Design review of the part built by this model. Coordinates are the model's own, in mm. A direction names the side the tool comes from. Coordinates: 2 decimals unless noted, no trailing zeros. Write each loop counter-clockwise with the first axis right and the second up, starting at its lowest first coordinate (ties: lowest second). Pieces come first, ordered by that corner, then holes.
Q1. Add section C-C, the plane y = 6.5. Give the boundary of the cut face in (x, z) (3 decimals).
Q2. To check wall thickness, follow probe 1 along X at (y, z) = (0.4, -12.1); probe 2 along X at (y, z) = (-1, -12.75); probe 3 along X at (y, z) = (2, -10.75). State the ranges of each line that lie inside material, in increasing order.
Q3. Add section D-D, the plane z = -8. Give the boundary of the cut face in (x, y).
Q4. The part is to be moulded in two halves that separate along X. For faces 1 (the face through (9.045, 1.521, -6.024)), 2 (the face through (-4, 2, -11)), 3 (the face through (9.5, 1.5, -7)), say which applies: +X half, -X half, draft (parallel to the pull), parting line (faces both ways), or undercut.
Q5. Add section A-A, the plane z = -5. Give the boundary of the cut face in (x, y) (3 decimals).
Q6. Clearance check with flat-ended pins moving along their axes: pin 1 Ø1.7 at (x, z) = (4, -4.5) entering from -Y; pin 2 Ø3.5 at (x, z) = (-1.5, -13) entering from -Y; pin 3 Ø1.7 at (y, z) = (7, -5.5) entering from +X; pin 4 Ø1.8 at (x, y) = (4, 7) entering from -Z. State where each tip first meets the part, or that it passes through.
Q7. Machinability: for faces 4 (the face through (5, 9.55, -5)), 5 (the face through (3, 6, -3)), 6 (the face through (-1.134, -0.021, -13.578)), 7 (the face through (-3.754, 0.305, -12.941)), 8 (the face through (1.45, 3.64, -14.2)), which of the approach directions +Z, -Z, +X, -X, +Y, -Y give a long, thin tool a straight path to every point of the face, cutting with its end or side? Answer none if there is none.
from build123d import *

# Parameters (mm, degrees)
SKETCH1_W           = 9
SKETCH1_H           = 9
BOSS_EXTRUDE1_DEPTH = 3
SKETCH2_W           = 2.95
SKETCH2_H           = 6
BOSS_EXTRUDE2_DEPTH = 6.1
FILLET1_R           = 3
SKETCH3_R           = 0.975
CUT_EXTRUDE1_DEPTH  = 11.1
CUT_EXTRUDE3_DEPTH  = 21.1
BOSS_EXTRUDE3_START = 4
SKETCH5_R           = 3
BOSS_EXTRUDE3_DEPTH = 4
SKETCH8_R           = 1.55
CUT_EXTRUDE4_DEPTH  = 3
CUT_EXTRUDE5_DEPTH  = 0.5
SKETCH10_W          = 9
SKETCH10_H          = 3
BOSS_EXTRUDE4_DEPTH = 4
SKETCH11_R          = 1
CUT_EXTRUDE6_DEPTH  = 4
CUT_EXTRUDE7_DEPTH  = 4
SKETCH13_W          = 6.1
SKETCH13_H          = 4
BOSS_EXTRUDE7_DEPTH = 7.5
SKETCH16_W          = 1.55
SKETCH16_H          = 4.1
CUT_EXTRUDE9_DEPTH  = 3.2
SKETCH17_W          = 4
SKETCH17_H          = 3
BOSS_EXTRUDE8_DEPTH = 2
SKETCH19_R          = 1.025
CUT_EXTRUDE10_DEPTH = 4
FILLET2_R           = 1


with BuildPart() as part:
    # Sketch1 → Boss-Extrude1 (new body)
    with BuildSketch(Plane(origin=(0, 0, 0), x_dir=(1, 0, 0), z_dir=(0, 1, 0))):
        with Locations((4.5, 4.5)):
            Rectangle(SKETCH1_W, SKETCH1_H)
    extrude(amount=BOSS_EXTRUDE1_DEPTH)

    # Sketch2 → Boss-Extrude2 (add)
    with BuildSketch(Plane(origin=(0, 0, -9), x_dir=(-1, 0, 0), z_dir=(0, 0, -1))):
        with Locations((-7.525, 1.5)):
            Rectangle(SKETCH2_W, SKETCH2_H)
        with Locations((-1.475, 1.5)):
            Rectangle(SKETCH2_W, SKETCH2_H)
    extrude(amount=BOSS_EXTRUDE2_DEPTH)

    # Fillet1
    fillet1_edges = [part.edges().sort_by_distance(p)[0] for p in [
        (1.475, 4.5, -15.1),
        (1.475, -1.5, -15.1),
        (7.525, -1.5, -15.1),
        (7.525, 4.5, -15.1),
    ]]
    fillet(fillet1_edges, radius=FILLET1_R - 0.0001)  # a hair under: the kernel refuses the full size

    # Sketch3 → Cut-Extrude1 (cut)
    with BuildSketch(Plane(origin=(9, 0, 0), x_dir=(0, 0, -1), z_dir=(1, 0, 0))):
        with Locations((12.1, 1.5)):
            Circle(SKETCH3_R)
    extrude(amount=-CUT_EXTRUDE1_DEPTH, mode=Mode.SUBTRACT)

    # Sketch6 → Cut-Extrude3 (cut)
    with BuildSketch(Plane.ZY):
        with BuildLine():
            Line((-12.1, 4.5), (-9, 4.5))
            Line((-9, 4.5), (-9, 3))
            Line((-9, 3), (-9.501923789, 3))
            ThreePointArc((-9.501923789, 3), (-10.6, 4.098076211), (-12.1, 4.5))
        make_face()
        with BuildLine():
            Line((-12.1, -1.5), (-9, -1.5))
            Line((-9, -1.5), (-9, 0))
            Line((-9, 0), (-9.501923789, 0))
            ThreePointArc((-9.501923789, 0), (-10.6, -1.098076211), (-12.1, -1.5))
        make_face()
    extrude(amount=-CUT_EXTRUDE3_DEPTH, mode=Mode.SUBTRACT)

    # Sketch5 → Boss-Extrude3 (add)
    with BuildSketch(Plane.ZY.offset(BOSS_EXTRUDE3_START)):
        with Locations((-12.1, 1.5)):
            Circle(SKETCH5_R)
    extrude(amount=-BOSS_EXTRUDE3_DEPTH)

    # Sketch8 → Cut-Extrude4 (cut)
    with BuildSketch(Plane(origin=(0, -1.5, 0), x_dir=(-1, 0, 0), z_dir=(0, -1, 0))):
        with Locations(Location((1.6, 12.1, 0), (0, 0, 90))):
            Circle(SKETCH8_R)
    extrude(amount=-CUT_EXTRUDE4_DEPTH, mode=Mode.SUBTRACT)

    # Sketch9 → Cut-Extrude5 (cut)
    with BuildSketch(Plane.ZY.offset(4)):
        with BuildLine():
            Line((-11.85, 1.5), (-11.85, -0.8))
            ThreePointArc((-11.85, -0.8), (-12.1, -1.05), (-12.35, -0.8))
            Line((-12.35, -0.8), (-12.35, 0.896446609))
            Line((-12.35, 0.896446609), (-13.549568901, -0.303122292))
            ThreePointArc((-13.549568901, -0.303122292), (-13.903122292, -0.303122292), (-13.903122292, 0.050431099))
            Line((-13.903122292, 0.050431099), (-12.703553391, 1.25))
            Line((-12.703553391, 1.25), (-14.4, 1.25))
            ThreePointArc((-14.4, 1.25), (-14.65, 1.5), (-14.4, 1.75))
            Line((-14.4, 1.75), (-12.703553391, 1.75))
            Line((-12.703553391, 1.75), (-13.903122292, 2.949568901))
            ThreePointArc((-13.903122292, 2.949568901), (-13.903122292, 3.303122292), (-13.549568901, 3.303122292))
            Line((-13.549568901, 3.303122292), (-12.35, 2.103553391))
            Line((-12.35, 2.103553391), (-12.35, 3.8))
            ThreePointArc((-12.35, 3.8), (-12.1, 4.05), (-11.85, 3.8))
            Line((-11.85, 3.8), (-11.85, 1.5))
        make_face()
    extrude(amount=-CUT_EXTRUDE5_DEPTH, mode=Mode.SUBTRACT)

    # Sketch10 → Boss-Extrude4 (add)
    with BuildSketch(Plane.XY):
        with Locations((4.5, 1.5)):
            Rectangle(SKETCH10_W, SKETCH10_H)
    extrude(amount=BOSS_EXTRUDE4_DEPTH)

    # Sketch11 → Cut-Extrude6 (cut)
    with BuildSketch(Plane(origin=(0, 3, 0), x_dir=(1, 0, 0), z_dir=(0, 1, 0))):
        with Locations(Location((4.5, -1, 0), (0, 0, 270))):
            Circle(SKETCH11_R)
    extrude(amount=-CUT_EXTRUDE6_DEPTH, mode=Mode.SUBTRACT)

    # Sketch12 → Cut-Extrude7 (cut)
    with BuildSketch(Plane(origin=(0, 3, 0), x_dir=(1, 0, 0), z_dir=(0, 1, 0))):
        with BuildLine():
            add(Edge.make_bspline(
                [(1.5, -1), (1.53988428, 0.555027292), (0.235256098, 1.545486909), (0, 3)],
                knots=[0, 0, 0, 0, 1, 1, 1, 1], degree=3))
            Line((0, 3), (0, -4))
            Line((0, -4), (4.5, -4))
            ThreePointArc((4.5, -4), (2.378679656, -3.121320344), (1.5, -1))
        make_face()
        with BuildLine():
            ThreePointArc((7.5, -1), (6.621320344, -3.121320344), (4.5, -4))
            Line((4.5, -4), (9, -4))
            Line((9, -4), (9, 3))
            add(Edge.make_bspline(
                [(7.5, -1), (7.46011572, 0.555027292), (8.764743902, 1.545486909), (9, 3)],
                knots=[0, 0, 0, 0, 1, 1, 1, 1], degree=3))
        make_face()
    extrude(amount=-CUT_EXTRUDE7_DEPTH, mode=Mode.SUBTRACT)

    # Sketch13 → Boss-Extrude7 (add)
    with BuildSketch(Plane(origin=(0, 3, 0), x_dir=(1, 0, 0), z_dir=(0, 1, 0))):
        with Locations((3.05, 5)):
            Rectangle(SKETCH13_W, SKETCH13_H)
    extrude(amount=BOSS_EXTRUDE7_DEPTH)

    # Sketch16 → Cut-Extrude9 (cut)
    with BuildSketch(Plane(origin=(6.1, 0, 0), x_dir=(0, 0, -1), z_dir=(1, 0, 0))):
        with Locations((5, 7.5)):
            Rectangle(SKETCH16_W, SKETCH16_H)
    extrude(amount=-CUT_EXTRUDE9_DEPTH, mode=Mode.SUBTRACT)

    # Sketch17 → Boss-Extrude8 (add)
    with BuildSketch(Plane(origin=(9, 0, 0), x_dir=(0, 0, -1), z_dir=(1, 0, 0))):
        with Locations((5, 1.5)):
            Rectangle(SKETCH17_W, SKETCH17_H)
    extrude(amount=BOSS_EXTRUDE8_DEPTH)

    # Sketch19 → Cut-Extrude10 (cut)
    with BuildSketch(Plane(origin=(0, 3, 0), x_dir=(1, 0, 0), z_dir=(0, 1, 0))):
        with Locations(Location((9, 5, 0), (0, 0, 270))):
            Circle(SKETCH19_R)
    extrude(amount=-CUT_EXTRUDE10_DEPTH, mode=Mode.SUBTRACT)

    # Fillet2
    fillet2_edges = [part.edges().sort_by_distance(p)[0] for p in [
        (0, 10.5, -5),
        (3.05, 10.5, -3),
        (3.05, 10.5, -7),
        (11, 1.5, -3),
        (11, 1.5, -7),
    ]]
    fillet(fillet2_edges, radius=FILLET2_R)


solid = part.part
Here are the results:
1. outline: (0, -7) - (6.1, -7) - (6.1, -5.775) - (2.9, -5.775) - (2.9, -4.225) - (6.1, -4.225) - (6.1, -3) - (0, -3) - close
2. probe 1: x = -3.5 to -3.15, -0.05 to 2.95, 6.05 to 9
2. probe 2: x = -4 to -3.01, -0.19 to 2.95, 6.05 to 9
2. probe 3: x = -4 to 2.95, 6.05 to 9
3. outline: (0, 0) - (9, 0) - (9, 3) - (0, 3) - close
4. face 1: undercut
4. face 2: -X half
4. face 3: draft
5. outline: (0, 0) - (7.975, 0) - (7.975, 3) - (6.1, 3) - (6.1, 5.45) - (2.9, 5.45) - (2.9, 9.55) - (6.1, 9.55) - (6.1, 10.5) - (1, 10.5) arc R1 ccw to (0, 9.5) - close; (10.025, 0) - (11, 0) - (11, 3) - (10.025, 3) - close
6. pin 1: stops at y = 0
6. pin 2: stops at y = -1.5
6. pin 3: stops at x = 6.1
6. pin 4: stops at z = -7
7. face 4: +X
7. face 5: +Z, +X, -X, +Y
7. face 6: -Y
7. face 7: -X
7. face 8: -Z, +X, -X, +Y
